Source: CAD feature listing. Evaluate the final solid. Frame: model axes, mm. A direction names the side the tool comes from. Round coordinates to 2 decimals unless told otherwise and drop trailing zeros. Write each loop counter-clockwise with the first axis right and the second up, starting at its lowest first coordinate (ties: lowest second). Pieces come first, ordered by that corner, then holes. Notation, with made-up numbers: M 78.5,13 L 132.5,13 A20 cw 132.5,25 Z; hole C 18,4.5 d8. An arc over 180 degrees is marked long. Use a Markdown table: item, result.
```python
from build123d import *

# Parameters (mm, degrees)
ESQUISSE1_R             = 13.75
BOSS_EXTRU_1_DEPTH      = 38
ESQUISSE2_W             = 11
ESQUISSE2_H             = 2
ENL_V_MAT_EXTRU_1_DEPTH = 14
BOSS_EXTRU_2_DEPTH      = 2
ESQUISSE5_R             = 8.5
BOSS_EXTRU_3_DEPTH      = 12
ESQUISSE6_R             = 9.5
BOSS_EXTRU_4_DEPTH      = 1


with BuildPart() as part:
    # Esquisse1 → Boss.-Extru.1 (new body)
    with BuildSketch(Plane.XY):
        Polygon((39.259818305, 17), (29.444863729, 34), (9.814954576, 34), (0, 17), (9.814954576, 0), (29.444863729, 0), align=None)
        with Locations((19.629909152, 17)):
            Circle(ESQUISSE1_R, mode=Mode.SUBTRACT)
    extrude(amount=BOSS_EXTRU_1_DEPTH)

    # Esquisse2 → Enlèv. mat.-Extru.1 (cut)
    with BuildSketch(Plane.XY.offset(38)):
        with Locations((19.629909152, 1)):
            Rectangle(ESQUISSE2_W, ESQUISSE2_H)
        Polygon((2.157477288, 13.263139721), (7.657477288, 3.736860279), (9.389528096, 4.736860279), (3.889528096, 14.263139721), align=None)
        Polygon((7.657477288, 30.263139721), (2.157477288, 20.736860279), (3.889528096, 19.736860279), (9.389528096, 29.263139721), align=None)
        with Locations((19.629909152, 33)):
            Rectangle(ESQUISSE2_W, ESQUISSE2_H)
        Polygon((37.102341017, 20.736860279), (31.602341017, 30.263139721), (29.870290209, 29.263139721), (35.370290209, 19.736860279), align=None)
        Polygon((31.602341017, 3.736860279), (37.102341017, 13.263139721), (35.370290209, 14.263139721), (29.870290209, 4.736860279), align=None)
    extrude(amount=-ENL_V_MAT_EXTRU_1_DEPTH, mode=Mode.SUBTRACT)

    # Esquisse4 → Boss.-Extru.2 (add)
    with BuildSketch(Plane(origin=(0, 0, 0), x_dir=(-1, 0, 0), z_dir=(0, 0, -1))):
        Polygon((-39.259818305, 17), (-29.444863729, 0), (-9.814954576, 0), (0, 17), (-9.814954576, 34), (-29.444863729, 34), align=None)
    extrude(amount=BOSS_EXTRU_2_DEPTH)

    # Esquisse5 → Boss.-Extru.3 (add)
    with BuildSketch(Plane(origin=(0, 0, -2), x_dir=(-1, 0, 0), z_dir=(0, 0, -1))):
        with Locations((-19.629909152, 17)):
            Circle(ESQUISSE5_R)
    extrude(amount=BOSS_EXTRU_3_DEPTH)

    # Esquisse6 → Boss.-Extru.4 (add)
    with BuildSketch(Plane(origin=(0, 0, -2), x_dir=(-1, 0, 0), z_dir=(0, 0, -1))):
        with Locations((-19.629909152, 17)):
            Circle(ESQUISSE6_R)
    extrude(amount=BOSS_EXTRU_4_DEPTH)


solid = part.part
```
Q1. Section D-D on y = 9.5. Return loops of the section in (x, z).
Results are:
| item | result |
|---|---|
| outline | M 4.33,-2 L 13.8,-2 L 13.8,-3 L 15.63,-3 L 15.63,-14 L 23.63,-14 L 23.63,-3 L 25.46,-3 L 25.46,-2 L 34.93,-2 L 34.93,24 L 32.62,24 L 32.62,38 L 31.15,38 L 31.15,0 L 8.11,0 L 8.11,38 L 6.64,38 L 6.64,24 L 4.33,24 Z |
Q2. Reachability of faces 1 (the flat face through (30.75, 29.77, 31.1)), 2 (the flat face through (20, 33, 24)), 3 (the cylindrical face through (11.78, 13.74, -8.42)) from +Z, -Z, +X, -X, +Y, -Y: full face, straight path, thin tool, end or side. Return the list, or none.
Results are:
| item | result |
|---|---|
| face 1 | +Z, +X |
| face 2 | +Z, +Y |
| face 3 | -Z |
Q3. Mould query, pull axis Y, two halves, no side actions, for faces 4 (the flat face through (36.248, 13.756, 31.098)), 5 (the flat face through (8.51, 4.23, 31.1)), 6 (the flat face through (4.84, 25.38, 13.84)). Classes: +Y half, -Y half, draft (parallel to the pull), parting line (faces both ways), or undercut.
Results are:
| item | result |
|---|---|
| face 4 | -Y half |
| face 5 | undercut |
| face 6 | +Y half |
Q4. First-contact query: pin 1 Ø1 at (x, z) = (33, 7.5) entering from +Y; pin 2 Ø2 at (y, z) = (33, 27.5) entering from -X; pin 3 Ø8 at (x, y) = (13, 15.5) entering from +Z. Flat tips, straight axial feed; report the tip coordinate or a pass-through.
Results are:
| item | result |
|---|---|
| pin 1 | y = 28.71 |
| pin 2 | x = 8.66 |
| pin 3 | z = 0 |
Q5. Section C-C on x = 17. Return loops of the section in (y, z).
Results are:
| item | result |
|---|---|
| outline | M 0,-2 L 7.87,-2 L 7.87,-3 L 8.92,-3 L 8.92,-14 L 25.08,-14 L 25.08,-3 L 26.13,-3 L 26.13,-2 L 34,-2 L 34,24 L 32,24 L 32,38 L 30.5,38 L 30.5,0 L 3.5,0 L 3.5,38 L 2,38 L 2,24 L 0,24 Z |
Q6. Line query: L1, parallel to Z at x = 30.5, y = 22.5; L2, parallel to Z at x = 24, y = 15; L3, parallel to Y at x = 29.5, z = 25.5. Output: solid intervals per line, ascending.
Results are:
| item | result |
|---|---|
| L1 | -2 to 0 |
| L2 | -14 to 0 |
| L3 | 0.1 to 7.43, 26.57 to 33.9 |
Q7. Section B-B on z = 3. Return loops of the section in (x, y).
Results are:
| item | result |
|---|---|
| outline | M 0,17 L 9.81,0 L 29.44,0 L 39.26,17 L 29.44,34 L 9.81,34 Z; hole C 19.63,17 d27.5 |
